Input: part model. Units: mm. Frame: model coordinates. Coordinates: 2 decimals unless noted, no trailing zeros. Loops run counter-clockwise (first coordinate to the right, second up) from the corner with the lowest first, then second, coordinate; pieces in that order, holes last. Notation, with made-up numbers: (-10, 21) - (48, 21) arc R24 ccw to (48, 48) - close; hole circle Ø1 at (86.5, -35.75). An arc over 180 degrees is marked (long way). Use a Markdown table: item, result. Add a question column.
1. Ray query, L1, parallel to X at y = -1.4, z = 83; L2, parallel to X at y = -0.95, z = 49.5; L3, parallel to Y at x = -224.5, z = 88. Return the intervals inside material, ascending. Write a range as [from, to].
2. Contact query for flat-ended pins moving along their axis: P1, Ø1, axis at y = -0.5, z = 57, coming from the -X side; P2, Ø3.5, axis at x = 89.5, z = -2, coming from the -Y side; P3, Ø1.6, axis at y = 0.5, z = -2, coming from the +X side. Output: stop coordinate, or through.
3. Section query D-D on z = 150. Return the cut outline in (x, y), then the cut area to 3 significant figures.
4. Section query A-A on z = 59. Return the cut outline in (x, y).
5. Section query C-C on x = -192. Return the cut outline in (y, z), then the cut area to 3 significant figures.
```python
from build123d import *

# Parameters (mm, degrees)
SKETCH1_W           = 457.2020066
SKETCH1_H           = 3.175
BOSS_EXTRUDE1_DEPTH = 200.6419914
SKETCH2_W           = 3.81
SKETCH2_H           = 114.3
CUT_EXTRUDE1_DEPTH  = 305.180387349
LPATTERN1_COUNT     = 4
LPATTERN1_PITCH     = 90.932
BOSS_EXTRUDE3_DEPTH = 3.175
SKETCH5_W           = 3.175
SKETCH5_H           = 88.392
CUT_EXTRUDE2_DEPTH  = 3.175
SKETCH3_W           = 49.658811606
SKETCH3_H           = 3.175
BOSS_EXTRUDE4_DEPTH = 3.175


with BuildPart() as part:
    # Sketch1 → Boss-Extrude1 (new body)
    with BuildSketch(Plane.XY):
        Rectangle(SKETCH1_W, SKETCH1_H)
    extrude(amount=BOSS_EXTRUDE1_DEPTH)

    # Sketch2 → Cut-Extrude1 (cut, through all)
    with BuildSketch(Plane(origin=(0, 1.5875, 0), x_dir=(1, 0, 0), z_dir=(0, 1, 0))):
        with Locations((135.8910033, -57.15)):
            Rectangle(SKETCH2_W, SKETCH2_H)
    cut_extrude1 = extrude(amount=-CUT_EXTRUDE1_DEPTH, mode=Mode.SUBTRACT)

    # LPattern1: Cut-Extrude1 ×4
    with Locations(*[(-i * LPATTERN1_PITCH, 0, 0) for i in range(1, LPATTERN1_COUNT)]):
        add(cut_extrude1, mode=Mode.SUBTRACT)

    # Sketch4 → Boss-Extrude3 (add)
    with BuildSketch(Plane.XZ.offset(1.5875)):
        Polygon((-228.6010033, 0), (-266.7010033, 0), (-228.6010033, 50.8), align=None)
    boss_extrude3 = extrude(amount=-BOSS_EXTRUDE3_DEPTH)

    # Mirror1: Boss-Extrude3 across plane
    add(boss_extrude3.mirror(Plane(origin=(0, 0, 0), x_dir=(0, 0, 1), z_dir=(1, 0, 0))))

    # Sketch5 → Cut-Extrude2 (cut)
    with BuildSketch(Plane.XZ.offset(1.5875)):
        with Locations((-227.0135033, 156.4459914)):
            Rectangle(SKETCH5_W, SKETCH5_H)
    cut_extrude2 = extrude(amount=-CUT_EXTRUDE2_DEPTH, mode=Mode.SUBTRACT)

    # Mirror2: Cut-Extrude2 across plane
    add(cut_extrude2.mirror(Plane(origin=(0, 0, 0), x_dir=(0, 0, 1), z_dir=(1, 0, 0))), mode=Mode.SUBTRACT)

    # Sketch3 → Boss-Extrude4 (add)
    with BuildSketch(Plane(origin=(0, 0, 0), x_dir=(-1, 0, 0), z_dir=(0, 0, -1))):
        with Locations((-91.020094169, 0.029240406)):
            Rectangle(SKETCH3_W, SKETCH3_H)
        with Locations((91.020094169, 0.029240406)):
            Rectangle(SKETCH3_W, SKETCH3_H)
    extrude(amount=BOSS_EXTRUDE4_DEPTH)


solid = part.part
```
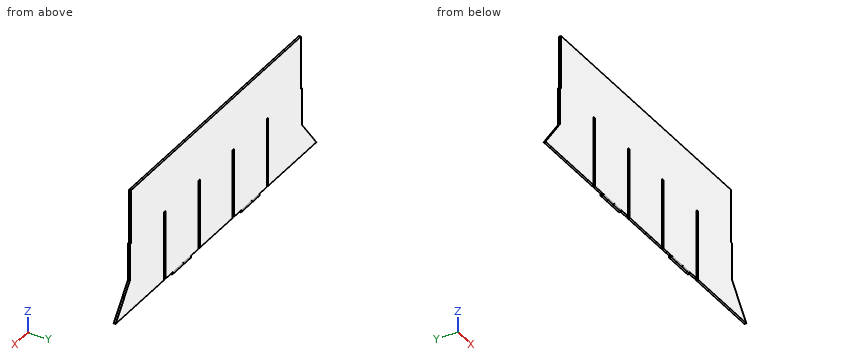
Resolved:
| question | item | result |
|---|---|---|
| 1 | L1 | [-228.6, -138.81], [-135, -47.88], [-44.07, 43.05], [46.86, 133.99], [137.8, 228.6] |
| 1 | L2 | [-229.58, -138.81], [-135, -47.88], [-44.07, 43.05], [46.86, 133.99], [137.8, 229.58] |
| 1 | L3 | [-1.59, 1.59] |
| 2 | P1 | x = -228.6 |
| 2 | P2 | y = -1.56 |
| 2 | P3 | x = 115.85 |
| 3 | outline | (-225.43, -1.59) - (225.43, -1.59) - (225.43, 1.59) - (-225.43, 1.59) - close |
| 3 | area | 1,430 mm² |
| 4 | outline | (-228.6, -1.59) - (-138.81, -1.59) - (-138.81, 1.59) - (-228.6, 1.59) - close; (-135, -1.59) - (-47.88, -1.59) - (-47.88, 1.59) - (-135, 1.59) - close; (-44.07, -1.59) - (43.05, -1.59) - (43.05, 1.59) - (-44.07, 1.59) - close; (46.86, -1.59) - (133.99, -1.59) - (133.99, 1.59) - (46.86, 1.59) - close; (137.8, -1.59) - (228.6, -1.59) - (228.6, 1.59) - (137.8, 1.59) - close |
| 5 | outline | (-1.59, 0) - (1.59, 0) - (1.59, 200.64) - (-1.59, 200.64) - close |
| 5 | area | 637 mm² |
